Design review of the part built by this model. Coordinates are the model's own, in mm. A direction names the side the tool comes from. Give positions to 0.01 mm unless a question says otherwise; leave off trailing zeros. Write each loop counter-clockwise with the first axis right and the second up, starting at its lowest first coordinate (ties: lowest second). Pieces come first, ordered by that corner, then holes. Notation, with made-up numbers: M -35,56.5 L -13,56.5 A22 ccw -13,63.5 Z; hole C 52.5,-28 d8. An arc over 180 degrees is marked long. Answer in a Markdown table with one row per item.
```python
from build123d import *

# Parameters (mm, degrees)
SKETCH1_R                = 250
BOSS_EXTRUDE1_DEPTH      = 10
CUT_EXTRUDE1_DEPTH       = 354.694783677
FILLET1_R                = 5
CIRPATTERN1_COUNT        = 7
FILLET1_OF_CIRPATTERN1_R = 5
SKETCH3_R                = 10
BOSS_EXTRUDE2_DEPTH      = 24.1
CHAMFER1_SIZE            = 1


with BuildPart() as part:
    # Sketch1 → Boss-Extrude1 (new body)
    with BuildSketch(Plane(origin=(0, 0, 0), x_dir=(1, 0, 0), z_dir=(0, 1, 0))):
        with Locations(Location((0, 0, 0), (0, 0, 270))):
            Circle(SKETCH1_R)
    extrude(amount=BOSS_EXTRUDE1_DEPTH)

    # Sketch2 → Cut-Extrude1 (cut, through all)
    with BuildSketch(Plane(origin=(0, 10, 0), x_dir=(1, 0, 0), z_dir=(0, 1, 0))):
        with BuildLine():
            Line((0, 15), (0, 200))
            ThreePointArc((0, 200), (68.404028665, 187.938524157), (128.557521937, 153.208888624))
            Line((128.557521937, 153.208888624), (9.641814145, 11.490666647))
            ThreePointArc((9.641814145, 11.490666647), (5.13030215, 14.095389312), (0, 15))
        make_face()
    cut_extrude1 = extrude(amount=-CUT_EXTRUDE1_DEPTH, mode=Mode.SUBTRACT)

    # Fillet1
    fillet1_edges = [part.edges().sort_by_distance(p)[0] for p in [
        (9.641814145, 5, -11.490666647),
        (0, 5, -15),
        (0, 5, -200),
        (128.557521937, 5, -153.208888624),
    ]]
    fillet(fillet1_edges, radius=FILLET1_R)

    # CirPattern1: Cut-Extrude1 ×7 about axis
    cirpattern1_axis = Axis((0, 0, 0), (0, 1, 0))
    for i in range(1, CIRPATTERN1_COUNT):
        add(cut_extrude1.rotate(cirpattern1_axis, i * 360 / CIRPATTERN1_COUNT), mode=Mode.SUBTRACT)

    # Fillet1 of CirPattern1
    fillet1_of_cirpattern1_edges = [part.edges().sort_by_distance(p)[0] for p in [
        (-2.972192148, 5, -14.702587318),
        (-11.727472237, 5, -9.352347028),
        (-156.366296494, 5, -124.697960372),
        (-39.62922864, 5, -196.03449757),
        (-13.348077132, 5, -6.84315986),
        (-14.623918683, 5, 3.337814009),
        (-194.985582436, 5, 44.504186791),
        (-177.974361762, 5, -91.242131471),
        (-13.672587785, 5, 6.169306547),
        (-6.508256087, 5, 13.514533019),
        (-86.776747824, 5, 180.19377358),
        (-182.301170462, 5, 82.257420626),
        (-3.701360965, 5, 14.536159293),
        (6.508256087, 5, 13.514533019),
        (86.776747824, 5, 180.19377358),
        (-49.351479538, 5, 193.815457246),
        (9.057066155, 5, 11.956987608),
        (14.623918683, 5, 3.337814009),
        (194.985582436, 5, 44.504186791),
        (120.760882065, 5, 159.426501445),
        (14.99533773, 5, 0.373960376),
        (11.727472237, 5, -9.352347028),
        (156.366296494, 5, -124.697960372),
        (199.9378364, 5, 4.986138348),
    ]]
    fillet(fillet1_of_cirpattern1_edges, radius=FILLET1_OF_CIRPATTERN1_R)

    # Sketch3 → Boss-Extrude2 (add)
    with BuildSketch(Plane(origin=(0, 10, 0), x_dir=(1, 0, 0), z_dir=(0, 1, 0))):
        with Locations(Location((0, 0, 0), (0, 0, 270))):
            Circle(SKETCH3_R)
    extrude(amount=BOSS_EXTRUDE2_DEPTH)

    # Chamfer1
    chamfer1_edges = [part.edges().sort_by_distance(p)[0] for p in [
        (0, 34.1, -10),
    ]]
    chamfer(chamfer1_edges, length=CHAMFER1_SIZE)


solid = part.part
```
1) Add section A-A (x = 184). Write out the cut boundary in (y, z), and give its area (3 significant figures).
Geometry says:
| item | result |
|---|---|
| outline | M 0,-169.25 L 10,-169.25 L 10,-78.38 L 0,-78.38 Z; M 0,4.59 L 10,4.59 L 10,42 L 0,42 Z; M 0,78.38 L 10,78.38 L 10,169.25 L 0,169.25 Z |
| area | 2,190 mm^2 |
2) Add section B-B (y = 27). Write out the cut boundary in (x, z), and give its area (3 significant figures).
Geometry says:
| item | result |
|---|---|
| outline | C 0,0 d20 |
| area | 314 mm^2 |
3) To check wall thickness, follow probe 1 along X at (y, z) = (5.5, -137.5); probe 2 along Z at (x, y) = (-70, 3); probe 3 along Z at (x, y) = (152, 8.5). State the ranges of each line that lie inside material, in increasing order. Write a range as [from, to].
Geometry says:
| item | result |
|---|---|
| probe 1 | [-208.79, -145.24], [-27.8, 0], [115.38, 208.79] |
| probe 2 | [-240, -187.35], [-55.82, -35.89], [15.98, 31.59], [145.36, 240] |
| probe 3 | [-198.48, -121.22], [3.79, 34.69], [129.98, 198.48] |
4) For faces 4 (the face through (4, 0, -3)), 5 (the face through (67.552, 5.07, -188.246)), list the 3-axis set-ups (+Z, -Z, +X, -X, +Y, -Y) from which the entire face can be reached by the end or side of a thin tool; tool diameter is ignored.
Geometry says:
| item | result |
|---|---|
| face 4 | +Z, -Z, +X, -X, -Y |
| face 5 | +Y, -Y |
5) Insertion check: P1, Ø8, axis at y = 4.5, z = -93, coming from the +X side; P2, Ø10, axis at y = 7, z = -67.5, coming from the +X side; P3, Ø4, axis at x = 96, y = 10.5, coming from the +Z side. Each pin has a flat end and moves straight along its axis. Give the tip position at first contact, or say it passes through.
Geometry says:
| item | result |
|---|---|
| P1 | x = 233.62 |
| P2 | x = 242.06 |
| P3 | z = 231.63 |
6) The part is to be moulded in two halves that separate along X. For faces 1 (the face through (-9.76, 21.39, -2.17)), 2 (the face through (0, 34.1, 0)), 3 (the face through (-142.54, 5.07, 140.294)), say which applies: released by +X, released by -X, zero draft, split by the parting line, or undercut.
Geometry says:
| item | result |
|---|---|
| face 1 | split by the parting line |
| face 2 | zero draft |
| face 3 | undercut |
